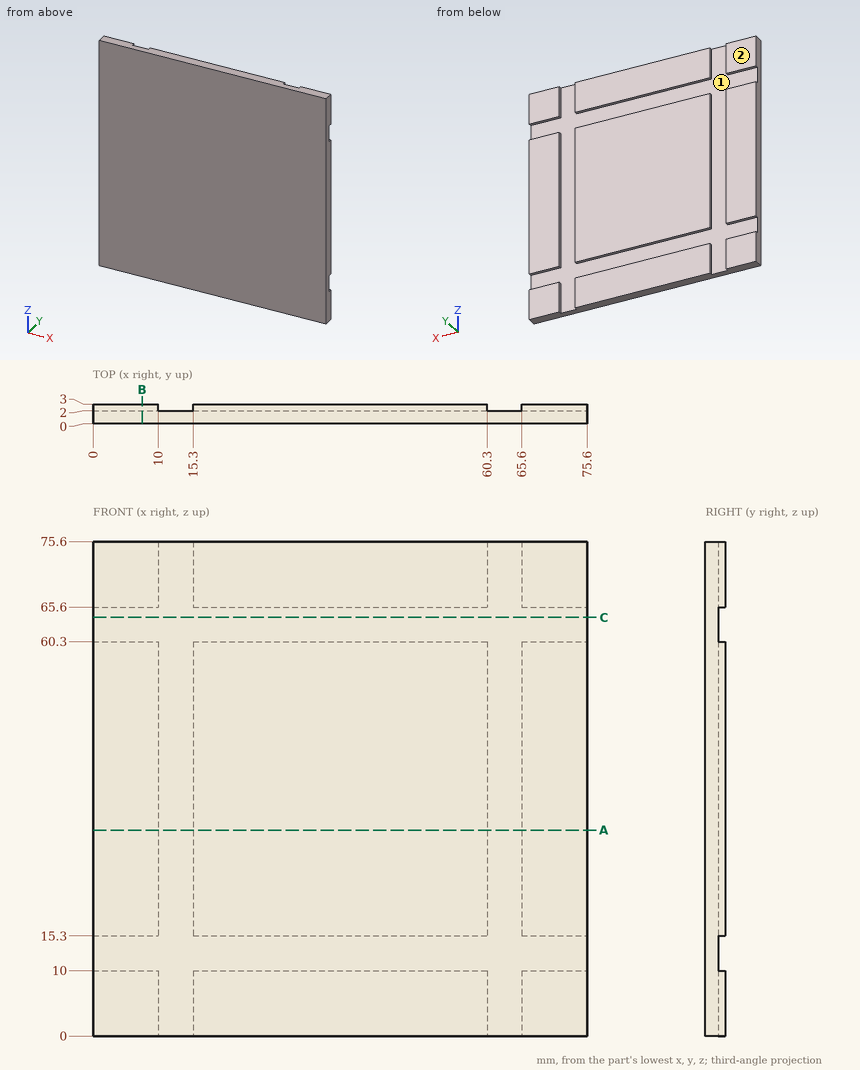
Can you work these out from the drawing? Everything is in mm from the part's minimum corner. Give positions to 0.01 mm unless a question says otherwise; leave off trailing zeros. Loops run counter-clockwise (first coordinate to the right, second up) from the corner with the lowest first, then second, coordinate; pieces in that order, holes last. Notation, with made-up numbers: (33.5, 23) - (67.5, 23) arc R10 ccw to (67.5, 28) - close; hole circle Ø10 at (-27.5, 48). An arc over 180 degrees is marked (long way). Use one line per item in the form item = value.
1. I need wall thicknesses on probe 1 along Z at (x, y) = (54.5, 2.1); probe 2 along Y at (x, z) = (10.5, 62). Which ranges of each line are inside material? Lowest first, please.
Response values:
probe_1 = 0 to 10, 15.3 to 60.3, 65.6 to 75.6
probe_2 = 0 to 2
2. I want a section at C-C (z = 64). Please give me the cut outline in (x, y), and give its area (3 significant figures).
Response values:
outline = (0, 0) - (75.6, 0) - (75.6, 2) - (0, 2) - close
area = 151 mm²
3. Thinking about a two-plate mould opening in Z: for the marked faces 1 and 2, which applies, released by +Z, released by -Z, zero draft, split by the parting line, or undercut?
Response values:
face_1 = undercut
face_2 = zero draft
4. I want a section at B-B (x = 7.5). Please give me the cut outline in (y, z), and give its area (3 significant figures).
Response values:
outline = (0, 0) - (3, 0) - (3, 10) - (2, 10) - (2, 15.3) - (3, 15.3) - (3, 60.3) - (2, 60.3) - (2, 65.6) - (3, 65.6) - (3, 75.6) - (0, 75.6) - close
area = 216 mm²
5. I'm going to push a flat-ended pin straight in: pin 1 Ø1.1 at (x, y) = (6.5, 2.5) entering from -Z. Where does the tip first touch, or does it pass through?
Response values:
pin_1 = 0
6. I want a section at A-A (z = 31.5). Please give me the cut outline in (x, y), and give its area (3 significant figures).
Response values:
outline = (0, 0) - (75.6, 0) - (75.6, 3) - (65.6, 3) - (65.6, 2) - (60.3, 2) - (60.3, 3) - (15.3, 3) - (15.3, 2) - (10, 2) - (10, 3) - (0, 3) - close
area = 216 mm²
